```python
from build123d import *

# Parameters (mm, degrees)
BOSS_EXTRUDE1_DEPTH = 20
SCALE1_SCALE        = 0.3
BOSS_EXTRUDE5_DEPTH = 12
BOSS_EXTRUDE2_DEPTH = 4
SKETCH5_R           = 6
BOSS_EXTRUDE3_DEPTH = 21
SKETCH10_W          = 7.23
SKETCH10_H          = 3.15
CUT_EXTRUDE1_DEPTH  = 12


with BuildPart() as part:
    # Sketch1 → Boss-Extrude1 (new, symmetric)
    with BuildSketch(Plane.XY.offset(19)):
        with BuildLine():
            Line((0, -23.5), (0, -29.5))
            Line((0, -29.5), (131.946891451, -29.5))
            Line((131.946891451, -29.5), (131.946891451, -23.5))
            Line((131.946891451, -23.5), (131.636124479, -23.5))
            ThreePointArc((131.636124479, -23.5), (131.349336261, -23.409576022), (131.166278168, -23.171010072))
            Line((131.166278168, -23.171010072), (129.648154655, -19))
            Line((129.648154655, -19), (127.962442939, -19))
            Line((127.962442939, -19), (126.444319426, -23.171010072))
            ThreePointArc((126.444319426, -23.171010072), (126.261261334, -23.409576022), (125.974473116, -23.5))
            Line((125.974473116, -23.5), (125.352939172, -23.5))
            ThreePointArc((125.352939172, -23.5), (125.066150953, -23.409576022), (124.883092861, -23.171010072))
            Line((124.883092861, -23.171010072), (123.364969348, -19))
            Line((123.364969348, -19), (121.679257632, -19))
            Line((121.679257632, -19), (120.161134119, -23.171010072))
            ThreePointArc((120.161134119, -23.171010072), (119.978076027, -23.409576022), (119.691287808, -23.5))
            Line((119.691287808, -23.5), (119.069753864, -23.5))
            ThreePointArc((119.069753864, -23.5), (118.782965646, -23.409576022), (118.599907554, -23.171010072))
            Line((118.599907554, -23.171010072), (117.081784041, -19))
            Line((117.081784041, -19), (115.396072325, -19))
            Line((115.396072325, -19), (113.877948812, -23.171010072))
            ThreePointArc((113.877948812, -23.171010072), (113.694890719, -23.409576022), (113.408102501, -23.5))
            Line((113.408102501, -23.5), (112.786568557, -23.5))
            ThreePointArc((112.786568557, -23.5), (112.499780339, -23.409576022), (112.316722247, -23.171010072))
            Line((112.316722247, -23.171010072), (110.798598734, -19))
            Line((110.798598734, -19), (109.112887017, -19))
            Line((109.112887017, -19), (107.594763504, -23.171010072))
            ThreePointArc((107.594763504, -23.171010072), (107.411705412, -23.409576022), (107.124917194, -23.5))
            Line((107.124917194, -23.5), (106.50338325, -23.5))
            ThreePointArc((106.50338325, -23.5), (106.216595032, -23.409576022), (106.03353694, -23.171010072))
            Line((106.03353694, -23.171010072), (104.515413427, -19))
            Line((104.515413427, -19), (102.82970171, -19))
            Line((102.82970171, -19), (101.311578197, -23.171010072))
            ThreePointArc((101.311578197, -23.171010072), (101.128520105, -23.409576022), (100.841731887, -23.5))
            Line((100.841731887, -23.5), (100.220197943, -23.5))
            ThreePointArc((100.220197943, -23.5), (99.933409725, -23.409576022), (99.750351632, -23.171010072))
            Line((99.750351632, -23.171010072), (98.23222812, -19))
            Line((98.23222812, -19), (96.546516403, -19))
            Line((96.546516403, -19), (95.02839289, -23.171010072))
            ThreePointArc((95.02839289, -23.171010072), (94.845334798, -23.409576022), (94.55854658, -23.5))
            Line((94.55854658, -23.5), (93.937012636, -23.5))
            ThreePointArc((93.937012636, -23.5), (93.650224417, -23.409576022), (93.467166325, -23.171010072))
            Line((93.467166325, -23.171010072), (91.949042812, -19))
            Line((91.949042812, -19), (90.263331096, -19))
            Line((90.263331096, -19), (88.745207583, -23.171010072))
            ThreePointArc((88.745207583, -23.171010072), (88.562149491, -23.409576022), (88.275361273, -23.5))
            Line((88.275361273, -23.5), (87.653827328, -23.5))
            ThreePointArc((87.653827328, -23.5), (87.36703911, -23.409576022), (87.183981018, -23.171010072))
            Line((87.183981018, -23.171010072), (85.665857505, -19))
            Line((85.665857505, -19), (83.980145789, -19))
            Line((83.980145789, -19), (82.462022276, -23.171010072))
            ThreePointArc((82.462022276, -23.171010072), (82.278964184, -23.409576022), (81.992175965, -23.5))
            Line((81.992175965, -23.5), (81.370642021, -23.5))
            ThreePointArc((81.370642021, -23.5), (81.083853803, -23.409576022), (80.900795711, -23.171010072))
            Line((80.900795711, -23.171010072), (79.382672198, -19))
            Line((79.382672198, -19), (77.696960481, -19))
            Line((77.696960481, -19), (76.178836969, -23.171010072))
            ThreePointArc((76.178836969, -23.171010072), (75.995778876, -23.409576022), (75.708990658, -23.5))
            Line((75.708990658, -23.5), (75.087456714, -23.5))
            ThreePointArc((75.087456714, -23.5), (74.800668496, -23.409576022), (74.617610404, -23.171010072))
            Line((74.617610404, -23.171010072), (73.099486891, -19))
            Line((73.099486891, -19), (71.413775174, -19))
            Line((71.413775174, -19), (69.895651661, -23.171010072))
            ThreePointArc((69.895651661, -23.171010072), (69.712593569, -23.409576022), (69.425805351, -23.5))
            Line((69.425805351, -23.5), (68.804271407, -23.5))
            ThreePointArc((68.804271407, -23.5), (68.517483189, -23.409576022), (68.334425097, -23.171010072))
            Line((68.334425097, -23.171010072), (66.816301584, -19))
            Line((66.816301584, -19), (65.130589867, -19))
            Line((65.130589867, -19), (63.612466354, -23.171010072))
            ThreePointArc((63.612466354, -23.171010072), (63.429408262, -23.409576022), (63.142620044, -23.5))
            Line((63.142620044, -23.5), (62.5210861, -23.5))
            ThreePointArc((62.5210861, -23.5), (62.234297882, -23.409576022), (62.051239789, -23.171010072))
            Line((62.051239789, -23.171010072), (60.533116276, -19))
            Line((60.533116276, -19), (58.84740456, -19))
            Line((58.84740456, -19), (57.329281047, -23.171010072))
            ThreePointArc((57.329281047, -23.171010072), (57.146222955, -23.409576022), (56.859434737, -23.5))
            Line((56.859434737, -23.5), (56.237900793, -23.5))
            ThreePointArc((56.237900793, -23.5), (55.951112574, -23.409576022), (55.768054482, -23.171010072))
            Line((55.768054482, -23.171010072), (54.249930969, -19))
            Line((54.249930969, -19), (52.564219253, -19))
            Line((52.564219253, -19), (51.04609574, -23.171010072))
            ThreePointArc((51.04609574, -23.171010072), (50.863037648, -23.409576022), (50.576249429, -23.5))
            Line((50.576249429, -23.5), (49.954715485, -23.5))
            ThreePointArc((49.954715485, -23.5), (49.667927267, -23.409576022), (49.484869175, -23.171010072))
            Line((49.484869175, -23.171010072), (47.966745662, -19))
            Line((47.966745662, -19), (46.281033946, -19))
            Line((46.281033946, -19), (44.762910433, -23.171010072))
            ThreePointArc((44.762910433, -23.171010072), (44.57985234, -23.409576022), (44.293064122, -23.5))
            Line((44.293064122, -23.5), (43.671530178, -23.5))
            ThreePointArc((43.671530178, -23.5), (43.38474196, -23.409576022), (43.201683868, -23.171010072))
            Line((43.201683868, -23.171010072), (41.683560355, -19))
            Line((41.683560355, -19), (39.997848638, -19))
            Line((39.997848638, -19), (38.479725125, -23.171010072))
            ThreePointArc((38.479725125, -23.171010072), (38.296667033, -23.409576022), (38.009878815, -23.5))
            Line((38.009878815, -23.5), (37.388344871, -23.5))
            ThreePointArc((37.388344871, -23.5), (37.101556653, -23.409576022), (36.918498561, -23.171010072))
            Line((36.918498561, -23.171010072), (35.400375048, -19))
            Line((35.400375048, -19), (33.714663331, -19))
            Line((33.714663331, -19), (32.196539818, -23.171010072))
            ThreePointArc((32.196539818, -23.171010072), (32.013481726, -23.409576022), (31.726693508, -23.5))
            Line((31.726693508, -23.5), (31.105159564, -23.5))
            ThreePointArc((31.105159564, -23.5), (30.818371346, -23.409576022), (30.635313253, -23.171010072))
            Line((30.635313253, -23.171010072), (29.117189741, -19))
            Line((29.117189741, -19), (27.431478024, -19))
            Line((27.431478024, -19), (25.913354511, -23.171010072))
            ThreePointArc((25.913354511, -23.171010072), (25.730296419, -23.409576022), (25.443508201, -23.5))
            Line((25.443508201, -23.5), (24.821974257, -23.5))
            ThreePointArc((24.821974257, -23.5), (24.535186039, -23.409576022), (24.352127946, -23.171010072))
            Line((24.352127946, -23.171010072), (22.834004433, -19))
            Line((22.834004433, -19), (21.148292717, -19))
            Line((21.148292717, -19), (19.630169204, -23.171010072))
            ThreePointArc((19.630169204, -23.171010072), (19.447111112, -23.409576022), (19.160322894, -23.5))
            Line((19.160322894, -23.5), (18.53878895, -23.5))
            ThreePointArc((18.53878895, -23.5), (18.252000731, -23.409576022), (18.068942639, -23.171010072))
            Line((18.068942639, -23.171010072), (16.550819126, -19))
            Line((16.550819126, -19), (14.86510741, -19))
            Line((14.86510741, -19), (13.346983897, -23.171010072))
            ThreePointArc((13.346983897, -23.171010072), (13.163925805, -23.409576022), (12.877137586, -23.5))
            Line((12.877137586, -23.5), (12.255603642, -23.5))
            ThreePointArc((12.255603642, -23.5), (11.968815424, -23.409576022), (11.785757332, -23.171010072))
            Line((11.785757332, -23.171010072), (10.267633819, -19))
            Line((10.267633819, -19), (8.581922103, -19))
            Line((8.581922103, -19), (7.06379859, -23.171010072))
            ThreePointArc((7.06379859, -23.171010072), (6.880740497, -23.409576022), (6.593952279, -23.5))
            Line((6.593952279, -23.5), (5.972418335, -23.5))
            ThreePointArc((5.972418335, -23.5), (5.685630117, -23.409576022), (5.502572025, -23.171010072))
            Line((5.502572025, -23.171010072), (3.984448512, -19))
            Line((3.984448512, -19), (2.298736795, -19))
            Line((2.298736795, -19), (0.780613282, -23.171010072))
            ThreePointArc((0.780613282, -23.171010072), (0.59755519, -23.409576022), (0.310766972, -23.5))
            Line((0.310766972, -23.5), (0, -23.5))
        make_face()
    extrude(amount=BOSS_EXTRUDE1_DEPTH, both=True)


with BuildPart() as part_1:
    # Scale1: scaled about (65.973445725, -25.112352152, 19)
    add(part.part.scale(SCALE1_SCALE).moved(Location((46.181412008, -17.578646506, 13.3))))

    # Sketch8 → Boss-Extrude5 (add)
    with BuildSketch(Plane.XY.offset(25)):
        Polygon((82.912250153, -26.428646507), (92.912250153, -26.428646507), (92.912250153, -7.428646507), align=None)
    extrude(amount=-BOSS_EXTRUDE5_DEPTH)

    # Sketch4 → Boss-Extrude2 (add)
    with BuildSketch(Plane(origin=(92.912250153, 0, 0), x_dir=(0, 0, -1), z_dir=(1, 0, 0))):
        Polygon((-13, -26.428646507), (-13, -14.428646507), (-13, -6.678646507), (-25, -6.678646507), (-25, -14.428646507), (-25, -26.428646507), align=None)
    extrude(amount=BOSS_EXTRUDE2_DEPTH)

    # Sketch5 → Boss-Extrude3 (add)
    with BuildSketch(Plane(origin=(96.912250153, 0, 0), x_dir=(0, 0, -1), z_dir=(1, 0, 0))):
        with Locations((-19, -14.428646507)):
            Circle(SKETCH5_R)
    extrude(amount=BOSS_EXTRUDE3_DEPTH)

    # Sketch10 → Cut-Extrude1 (cut)
    with BuildSketch(Plane.XY.offset(25)):
        with Locations((49.796412008, -24.853646507)):
            Rectangle(SKETCH10_W, SKETCH10_H)
    extrude(amount=-CUT_EXTRUDE1_DEPTH, mode=Mode.SUBTRACT)


solid = part_1.part
```
Input: part model. Units: mm. Frame: model coordinates. A direction names the side the tool comes from. Coordinates: 2 decimals unless noted, no trailing zeros. Write each loop counter-clockwise with the first axis right and the second up, starting at its lowest first coordinate (ties: lowest second). Pieces come first, ordered by that corner, then holes. Notation, with made-up numbers: (55.5, 62) - (76.5, 62) arc R23 cw to (76.5, 73) - close; hole circle Ø2 at (-18.75, 61). An arc over 180 degrees is marked (long way). Put each result on its own line as item: value. Start each with the question number.
1) Ray query, L1, parallel to X at y = -24.75, z = 19.5; L2, parallel to Y at x = 63, z = 21.25; L3, parallel to Y at x = 79, z = 14. Return the intervals inside material, ascending.
2) Cut plane C-C (y = -22.5). Return the cut outline in (x, z).
3) Reachability of faces 4 (the face through (58.917, -23.913, 19.084)), 5 (the face through (86, -21, 25)) from +Z, -Z, +X, -X, +Y, -Y: full face, straight path, thin tool, end or side. Return the list, or none.
4) Cut plane B-B (y = -16.75). Return the cut outline in (x, z), plus the area to 3 significant figures.
5) Cut plane A-A (y = -13.5). Return the cut outline in (x, z).
6) Contact query for flat-ended pins moving along their axis: pin 1 (5 mm diameter, centred on y = -11.5, z = 20.5, fed in from -X); pin 2 (1.5 mm diameter, centred on y = -23, z = 17.5, fed in from +X); pin 3 (0.6 mm diameter, centred on x = 77.5, z = 16, fed in from +Y); pin 4 (6 mm diameter, centred on x = 99.5, y = -11.5, fed in from +Z). Output: stop coordinate, or through.
7) Mould query, pull axis X, two halves, no side actions, for faces 1 (the face through (57.956, -23.896, 19.084)), 2 (the face through (96.912, -23, 19)), 3 (the face through (107.27, -8.48, 19.78)). Classes: pulls with the +X half, pulls with the -X half, needs draft (parallel to the pull), parting line crosses it, or undercut.
Resolved:
1. L1: x = 53.41 to 96.91
1. L2: y = -26.43 to -24.62
1. L3: y = -26.43 to -23.28
2. outline: (84.98, 13) - (96.91, 13) - (96.91, 25) - (84.98, 25) - close
3. face 4: +Z, -Z, +Y
3. face 5: +Z, +X, -X, +Y, -Y
4. outline: (88.01, 13) - (96.91, 13) - (96.91, 13.47) - (117.91, 13.47) - (117.91, 24.53) - (96.91, 24.53) - (96.91, 25) - (88.01, 25) - close
4. area: 339 mm2
5. outline: (89.72, 13) - (96.91, 13) - (96.91, 13.07) - (117.91, 13.07) - (117.91, 24.93) - (96.91, 24.93) - (96.91, 25) - (89.72, 25) - close
6. pin 1: stops at x = 89.45
6. pin 2: stops at x = 96.91
6. pin 3: stops at y = -23.28
6. pin 4: stops at z = 25
7. face 1: undercut
7. face 2: pulls with the +X half
7. face 3: needs draft
